Design review of the part built by this model. Coordinates are the model's own, in mm. A direction names the side the tool comes from. Round coordinates to 2 decimals unless told otherwise and drop trailing zeros. Use a Markdown table: item, result. Add a question column.
(1) For pin 1 (1.5 mm diameter, centred on x = -7.5, y = 1.5, fed in from -Z); pin 2 (1.6 mm diameter, centred on x = -31.5, y = 1, fed in from +Z); pin 3 (1.5 mm diameter, centred on y = 1.5, z = -41.5, fed in from +X), all flat-tipped, find the tip position at first contact; note any pin that passes through.
(2) Take a section at A-A (y = 1.25). Count the separate pieces of the cut face and the enclosed holes in it, then the cut area to 3 significant figures.
(3) Machinability: for faces 1 (the face through (0, 1, -43)), 2 (the face through (10, 1, -40)), 3 (the face through (75, 1, -40)), 4 (the face through (79.45, 1, -11)), 5 (the face through (-15, 1, -20)), which of the approach directions +Z, -Z, +X, -X, +Y, -Y give a long, thin tool a straight path to every point of the face, cutting with its end or side? Answer none if there is none.
(4) The part is to be moulded in two halves that separate along Z. For faces 6 (the face through (-10, 1, 0)), 7 (the face through (-39, 1, -20)), 8 (the face through (17, 1, -34)), say which applies: released by +Z, released by -Z, zero draft, split by the parting line, or undercut.
(5) To check wall thickness, follow probe 1 along Z at (x, y) = (-75, 1.95); probe 2 along X at (y, z) = (0.4, -40.5); probe 3 along Z at (x, y) = (38, 1.7). State the ranges of each line that lie inside material, in increasing order. Write a range as from..to.
```python
from build123d import *

# Parameters (mm, degrees)
SKETCH1_W           = 2
SKETCH1_H           = 36
SKETCH1_H_2         = 11
BOSS_EXTRUDE1_DEPTH = 3


with BuildPart() as part:
    # Sketch1 → Boss-Extrude1 (new body)
    with BuildSketch(Plane(origin=(0, 0, 0), x_dir=(1, 0, 0), z_dir=(0, 1, 0))):
        Polygon((-83, 40), (-79.45, 40), (-79.45, 32.5), (-81.25, 32.5), (-81.25, 30), (-79.45, 30), (-79.45, 27), (-76.55, 27), (-76.55, 30), (-74.75, 30), (-74.75, 32.5), (-76.55, 32.5), (-76.55, 40), (-73, 40), (-73, 43), (-63, 43), (-63, 40), (-49, 40), (-49, 27.5), (-47, 27.5), (-47, 40), (-41, 40), (-41, 27.5), (-39, 27.5), (-39, 40), (-33, 40), (-33, 27.5), (-31, 27.5), (-31, 40), (-25, 40), (-25, 27.5), (-23, 27.5), (-23, 40), (-17, 40), (-17, 27.5), (-15, 27.5), (-15, 40), (-5, 40), (-5, 43), (5, 43), (5, 40), (15, 40), (15, 27.5), (17, 27.5), (17, 40), (23, 40), (23, 27.5), (25, 27.5), (25, 40), (31, 40), (31, 27.5), (33, 27.5), (33, 40), (39, 40), (39, 27.5), (41, 27.5), (41, 40), (47, 40), (47, 27.5), (49, 27.5), (49, 40), (63, 40), (63, 43), (73, 43), (73, 40), (76.55, 40), (76.55, 32.5), (74.75, 32.5), (74.75, 30), (76.55, 30), (76.55, 27), (79.45, 27), (79.45, 30), (81.25, 30), (81.25, 32.5), (79.45, 32.5), (79.45, 40), (83, 40), (83, 0), (79.45, 0), (79.45, 7.5), (81.25, 7.5), (81.25, 10), (79.45, 10), (79.45, 13), (76.55, 13), (76.55, 10), (74.75, 10), (74.75, 7.5), (76.55, 7.5), (76.55, 0), (73, 0), (73, -3), (63, -3), (63, 0), (49, 0), (49, 12.5), (47, 12.5), (47, 0), (41, 0), (41, 12.5), (39, 12.5), (39, 0), (33, 0), (33, 12.5), (31, 12.5), (31, 0), (25, 0), (25, 12.5), (23, 12.5), (23, 0), (17, 0), (17, 12.5), (15, 12.5), (15, 0), (5, 0), (5, -3), (-5, -3), (-5, 0), (-15, 0), (-15, 12.5), (-17, 12.5), (-17, 0), (-23, 0), (-23, 12.5), (-25, 12.5), (-25, 0), (-31, 0), (-31, 12.5), (-33, 12.5), (-33, 0), (-39, 0), (-39, 12.5), (-41, 12.5), (-41, 0), (-47, 0), (-47, 12.5), (-49, 12.5), (-49, 0), (-63, 0), (-63, -3), (-73, -3), (-73, 0), (-76.55, 0), (-76.55, 7.5), (-74.75, 7.5), (-74.75, 10), (-76.55, 10), (-76.55, 13), (-79.45, 13), (-79.45, 10), (-81.25, 10), (-81.25, 7.5), (-79.45, 7.5), (-79.45, 0), (-83, 0), align=None)
        with Locations((-52, 20)):
            Rectangle(SKETCH1_W, SKETCH1_H, mode=Mode.SUBTRACT)
        with Locations((-44, 20)):
            Rectangle(SKETCH1_W, SKETCH1_H, mode=Mode.SUBTRACT)
        with Locations((-36, 20)):
            Rectangle(SKETCH1_W, SKETCH1_H, mode=Mode.SUBTRACT)
        with Locations((-28, 20)):
            Rectangle(SKETCH1_W, SKETCH1_H, mode=Mode.SUBTRACT)
        with Locations((-20, 20)):
            Rectangle(SKETCH1_W, SKETCH1_H, mode=Mode.SUBTRACT)
        with Locations((-48, 20)):
            Rectangle(SKETCH1_W, SKETCH1_H_2, mode=Mode.SUBTRACT)
        with Locations((-40, 20)):
            Rectangle(SKETCH1_W, SKETCH1_H_2, mode=Mode.SUBTRACT)
        with Locations((-32, 20)):
            Rectangle(SKETCH1_W, SKETCH1_H_2, mode=Mode.SUBTRACT)
        with Locations((-24, 20)):
            Rectangle(SKETCH1_W, SKETCH1_H_2, mode=Mode.SUBTRACT)
        with Locations((-16, 20)):
            Rectangle(SKETCH1_W, SKETCH1_H_2, mode=Mode.SUBTRACT)
        with Locations((16, 20)):
            Rectangle(SKETCH1_W, SKETCH1_H_2, mode=Mode.SUBTRACT)
        with Locations((20, 20)):
            Rectangle(SKETCH1_W, SKETCH1_H, mode=Mode.SUBTRACT)
        with Locations((24, 20)):
            Rectangle(SKETCH1_W, SKETCH1_H_2, mode=Mode.SUBTRACT)
        with Locations((28, 20)):
            Rectangle(SKETCH1_W, SKETCH1_H, mode=Mode.SUBTRACT)
        with Locations((32, 20)):
            Rectangle(SKETCH1_W, SKETCH1_H_2, mode=Mode.SUBTRACT)
        with Locations((36, 20)):
            Rectangle(SKETCH1_W, SKETCH1_H, mode=Mode.SUBTRACT)
        with Locations((40, 20)):
            Rectangle(SKETCH1_W, SKETCH1_H_2, mode=Mode.SUBTRACT)
        with Locations((48, 20)):
            Rectangle(SKETCH1_W, SKETCH1_H_2, mode=Mode.SUBTRACT)
        with Locations((44, 20)):
            Rectangle(SKETCH1_W, SKETCH1_H, mode=Mode.SUBTRACT)
        with Locations((52, 20)):
            Rectangle(SKETCH1_W, SKETCH1_H, mode=Mode.SUBTRACT)
    extrude(amount=BOSS_EXTRUDE1_DEPTH)


solid = part.part
```
Verdict:
| question | item | result |
|---|---|---|
| 1 | pin 1 | stops at z = -40 |
| 1 | pin 2 | stops at z = 0 |
| 1 | pin 3 | stops at x = 73 |
| 2 | separate pieces | 1 |
| 2 | enclosed holes | 20 |
| 2 | area | 5,190 mm^2 |
| 3 | face 1 | -Z, +X, -X, +Y, -Y |
| 3 | face 2 | -Z, +Y, -Y |
| 3 | face 3 | -Z, +X, +Y, -Y |
| 3 | face 4 | +Z, +Y, -Y |
| 3 | face 5 | +Y, -Y |
| 4 | face 6 | released by +Z |
| 4 | face 7 | undercut |
| 4 | face 8 | zero draft |
| 5 | probe 1 | z = -40..-32.5, -30..-10, -7.5..0 |
| 5 | probe 2 | x = -73..-63, -5..5, 63..73 |
| 5 | probe 3 | z = -40..0 |
